Autodesk Inventor part; units mm, degrees
ref_plane "YZ Plane" through (0, 0, 0) normal (1, 0, 0) x (0, 1, 0)
ref_plane "XZ Plane" through (0, 0, 0) normal (0, 1, 0) x (-1, 0, 0)
ref_plane "XY Plane" through (0, 0, 0) normal (0, 0, 1) x (1, 0, 0)
sketch "Sketch1" plane through (0, 0, 0) normal (0, 0, 1) x (1, 0, 0)
  arc A0 (-29.1377, 4.6094) -> (29.1377, 4.6094) centre (0, 0) ccw
  line L0 (-29.1377, 4.6094) -> (-34.1913, 4.6094)
  line L1 (29.1377, 4.6094) -> (34.281, 4.6755)
  line L2 (29.1377, 4.6094) -> (34.281, 4.6755) construction
  line L3 (5.3378, -34.5235) -> (5.3378, -49.5235)
  line L4 (5.3378, -49.5235) -> (-4.6622, -49.5235)
  line L5 (-4.6622, -49.5235) -> (-4.6622, -34.5235)
  line L6 (-4.6622, -34.5235) -> (-4.6622, -34.1841)
  line L7 (5.3378, -34.5235) -> (5.3378, -34.1841)
  arc A1 (-34.1913, 4.6094) -> (-4.6622, -34.1841) centre (0, 0) ccw
  arc A2 (5.3378, -34.1841) -> (34.281, 4.6755) centre (0, 0) ccw
  dimension "d0" = 59
  dimension "d5" = 10
  dimension "d6" = 15
extrude "Extrusion1" add sketch "Sketch1" along normal blind 5
properties part number "Clip_TestFitV1"
Here's how the part is built. I have some questions about the finished solid (model axes, mm). A direction names the side the tool comes from. Coordinates: 2 decimals unless noted, no trailing zeros. Order: outer loops, then holes, each group sorted by start corner. A loop starts at its lowest first (then second) coordinate and runs counter-clockwise, first axis right, second up.
Item 1: If we section it at D-D on y = -35: List the corners of the cut face in (x, z) for me.
Result sheet:
outline: (-4.66, 0) - (5.34, 0) - (5.34, 5) - (-4.66, 5) - close
Item 2: For faces 1 (the face through (-32, 4.609, 2)), 2 (the face through (0, -49.524, 2)), 3 (the face through (-4.662, -42, 2)), which set-ups out of +Z, -Z, +X, -X, +Y, -Y let a thin tool reach every point of the face, with its end or its side?
Result sheet:
face 1: +Z, -Z, -X, +Y
face 2: +Z, -Z, +X, -X, -Y
face 3: +Z, -Z, -X, -Y
Item 3: For P1, Ø1, axis at y = -19, z = 3, coming from the -X side; P2, Ø3, axis at x = 22, z = 3, coming from the +Y side; P3, Ø2.5, axis at y = -44, z = 2, coming from the +X side, each with a flat end and sliding along its axis, tell me the tip position at first contact or that it passes through.
Result sheet:
P1: stops at x = -29.12
P2: stops at y = -17.83
P3: stops at x = 5.34
Item 4: If we section it at C-C on x = 0: List the corners of the cut face in (y, z) for me, plus the area to 3 significant figures.
Result sheet:
outline: (-49.52, 0) - (-29.5, 0) - (-29.5, 5) - (-49.52, 5) - close
area: 100 mm2
Item 5: If we mould it in two halves opening along X, with no side actions, what happens to faces 4 (the face through (0, -30, 0)), 5 (the face through (0.71, -29.49, 2.46)), 6 (the face through (5.338, -42, 2)), 7 (the face through (-27.22, -21.2, 2.46))? For each: +X half, -X half, draft (parallel to the pull), parting line (faces both ways), or undercut.
Result sheet:
face 4: draft
face 5: undercut
face 6: +X half
face 7: -X half
Item 6: If we section it at B-B on z = 2.8: List the corners of the cut face in (x, y) for me, plus the area to 3 significant figures.
Result sheet:
outline: (-34.19, 4.61) arc R34.5 ccw to (-4.66, -34.18) - (-4.66, -49.52) - (5.34, -49.52) - (5.34, -34.18) arc R34.6 ccw to (34.28, 4.68) - (29.14, 4.61) arc R29.5 cw (long way) to (-29.14, 4.61) - close
area: 706 mm2
Item 7: I need wall thicknesses on line 1 (X direction, y = 0, z = 1.45); line 2 (X direction, y = -22.5, z = 2.95); line 3 (X direction, y = -44.5, z = 0.45). Which ranges of each line are inside material? Lowest first, please.
Result sheet:
line 1: x = -34.5 to -29.5, 29.5 to 34.6
line 2: x = -26.15 to -19.08, 19.08 to 26.28
line 3: x = -4.66 to 5.34
Item 8: If we section it at A-A on y = 0: List the corners of the cut face in (x, z) for me.
Result sheet:
outline: (-34.5, 0) - (-29.5, 0) - (-29.5, 5) - (-34.5, 5) - close; (29.5, 0) - (34.6, 0) - (34.6, 5) - (29.5, 5) - close
